from build123d import *

# Parameters (mm, degrees)
SALIENTE_EXTRUIR1_DEPTH = 2.5
CROQUIS2_W              = 5
CROQUIS2_H              = 12.7
SALIENTE_EXTRUIR2_DEPTH = 6.350000000000001
CORTAR_EXTRUIR1_REACH   = 52.655
CORTAR_EXTRUIR2_REACH   = 52.655
MATRIZC7_COUNT          = 3
REDONDEO3_R             = 3
REDONDEO4_R             = 3
REDONDEO5_R             = 3
REDONDEO6_R             = 3
REDONDEO7_R             = 3
REDONDEO8_R             = 3


with BuildPart() as part:
    # Croquis1 → Saliente-Extruir1 (new, symmetric)
    with BuildSketch(Plane(origin=(0, 0, 0), x_dir=(1, 0, 0), z_dir=(0, 1, 0))):
        with BuildLine():
            Line((-2.5, 28.650000000000002), (2.5, 28.650000000000002))
            Line((2.5, 28.650000000000002), (2.5, 20.849364905389077))
            ThreePointArc((2.5, 20.849364905389077), (2.8407417371092976, 18.26117445436386), (3.8397459621556003, 15.84936490538906))
            Line((3.8397459621556003, 15.84936490538906), (15.64582562299427, -4.599364905389191))
            ThreePointArc((15.64582562299427, -4.599364905389191), (17.235011848973173, -6.670432717254639), (19.306079660838602, -8.259618943233573))
            Line((19.306079660838602, -8.259618943233573), (26.061627818424082, -12.159936490539094))
            Line((26.061627818424082, -12.159936490539094), (23.561627818424125, -16.490063509461137))
            Line((23.561627818424125, -16.490063509461137), (16.806079660838638, -12.589745962155668))
            ThreePointArc((16.806079660838638, -12.589745962155668), (14.394270111863824, -11.590741737109344), (11.80607966083859, -11.25000000000002))
            Line((11.80607966083859, -11.25000000000002), (-11.806079660838877, -11.250000000000021))
            ThreePointArc((-11.806079660838877, -11.250000000000021), (-14.394270111864046, -11.590741737109328), (-16.806079660838808, -12.589745962155595))
            Line((-16.806079660838808, -12.589745962155595), (-23.561627818424295, -16.490063509460935))
            Line((-23.561627818424295, -16.490063509460935), (-26.061627818424316, -12.15993649053858))
            Line((-26.061627818424316, -12.15993649053858), (-19.30607966083857, -8.259618943233107))
            ThreePointArc((-19.30607966083857, -8.259618943233107), (-17.235011848973045, -6.670432717254254), (-15.645825622994131, -4.5993649053887635))
            Line((-15.645825622994131, -4.5993649053887635), (-3.8397459621555967, 15.849364905389269))
            ThreePointArc((-3.8397459621555967, 15.849364905389269), (-2.8407417371093064, 18.26117445436405), (-2.5000000000000004, 20.84936490538924))
            Line((-2.5000000000000004, 20.84936490538924), (-2.5, 28.650000000000002))
        make_face()
        with BuildLine():
            Line((4.999999999999967, -1.648e-14), (8.325317547305488, -1.919872981077918))
            Line((8.325317547305488, -1.919872981077918), (2.5, 8.169872981077836))
            Line((2.5, 8.169872981077836), (2.5000000000000004, 4.330127018922162))
            ThreePointArc((2.5000000000000004, 4.330127018922162), (3.16987298107781, 1.8301270189221883), (4.999999999999967, -1.648e-14))
        make_face(mode=Mode.SUBTRACT)
        with BuildLine():
            Line((-2.499999999999762, -4.330127018922147), (-5.825317547305628, -6.250000000000082))
            Line((-5.825317547305628, -6.250000000000082), (5.825317547305489, -6.249999999999961))
            Line((5.825317547305489, -6.249999999999961), (2.5000000000002185, -4.3301270189221945))
            ThreePointArc((2.5000000000002185, -4.3301270189221945), (1.9836e-13, -3.660254037844239), (-2.499999999999762, -4.330127018922147))
        make_face(mode=Mode.SUBTRACT)
        with BuildLine():
            Line((-2.5000000000000004, 4.330127018922227), (-2.5, 8.169872981077782))
            Line((-2.5, 8.169872981077782), (-8.325317547305644, -1.9198729810777775))
            Line((-8.325317547305644, -1.9198729810777775), (-5.000000000000053, 0))
            ThreePointArc((-5.000000000000053, 0), (-3.1698729810778152, 1.8301270189221972), (-2.5000000000000004, 4.330127018922227))
        make_face(mode=Mode.SUBTRACT)
    extrude(amount=SALIENTE_EXTRUIR1_DEPTH, both=True)

    # Croquis2 → Saliente-Extruir2 (add, symmetric)
    with BuildSketch(Plane(origin=(0, 0, 0), x_dir=(1, 0, 0), z_dir=(0, 1, 0))):
        with Locations((0, 35)):
            Rectangle(CROQUIS2_W, CROQUIS2_H)
    saliente_extruir2 = extrude(amount=SALIENTE_EXTRUIR2_DEPTH, both=True)

    # Croquis3 → Cortar-Extruir1 (cut, up to next)
    with BuildSketch(Plane(origin=(2.5, 0, 0), x_dir=(0, 0, -1), z_dir=(1, 0, 0)), mode=Mode.PRIVATE) as cortar_extruir1_sk1:
        with BuildLine():
            Line((32.754935969732706, 2.2450640302672804), (35, 4.490128060534589))
            Line((35, 4.490128060534589), (37.245064030267294, 2.245064030267292))
            ThreePointArc((37.245064030267294, 2.245064030267292), (35.00000000000001, -3.174999999999998), (32.754935969732706, 2.2450640302672804))
        make_face()
    cortar_extruir1_tool1 = extrude(cortar_extruir1_sk1.sketch, amount=-CORTAR_EXTRUIR1_REACH, mode=Mode.PRIVATE) & part.part
    cortar_extruir1 = cortar_extruir1_tool1.solids().sort_by_distance((2.5, 0.222977, -35))[0]
    add(cortar_extruir1, mode=Mode.SUBTRACT)

    # Croquis4 → Cortar-Extruir2 (cut, up to next)
    with BuildSketch(Plane.ZY.offset(2.5000000000000018), mode=Mode.PRIVATE) as cortar_extruir2_sk1:
        with BuildLine():
            Line((-41.35, 6.350000000000001), (-37.50000000000001, 6.350000000000001))
            ThreePointArc((-37.50000000000001, 6.350000000000001), (-40.22236110756822, 5.222361107568213), (-41.35, 2.500000000000002))
            Line((-41.35, 2.500000000000002), (-41.35, 6.350000000000001))
        make_face()
    cortar_extruir2_tool1 = extrude(cortar_extruir2_sk1.sketch, amount=-CORTAR_EXTRUIR2_REACH, mode=Mode.PRIVATE) & part.part
    # Croquis4 → Cortar-Extruir2 (cut, up to next)
    with BuildSketch(Plane.ZY.offset(2.5000000000000018), mode=Mode.PRIVATE) as cortar_extruir2_sk2:
        with BuildLine():
            Line((-32.5, 6.350000000000001), (-28.650000000000002, 6.350000000000001))
            Line((-28.650000000000002, 6.350000000000001), (-28.650000000000002, 2.5))
            ThreePointArc((-28.650000000000002, 2.5), (-29.777638892431792, 5.222361107568209), (-32.5, 6.350000000000001))
        make_face()
    cortar_extruir2_tool2 = extrude(cortar_extruir2_sk2.sketch, amount=-CORTAR_EXTRUIR2_REACH, mode=Mode.PRIVATE) & part.part
    # Croquis4 → Cortar-Extruir2 (cut, up to next)
    with BuildSketch(Plane.ZY.offset(2.5000000000000018), mode=Mode.PRIVATE) as cortar_extruir2_sk3:
        with BuildLine():
            Line((-41.35, -2.500000000000002), (-41.35, -6.350000000000001))
            Line((-41.35, -6.350000000000001), (-37.50000000000001, -6.350000000000001))
            ThreePointArc((-37.50000000000001, -6.350000000000001), (-40.22236110756821, -5.222361107568203), (-41.35, -2.500000000000002))
        make_face()
    cortar_extruir2_tool3 = extrude(cortar_extruir2_sk3.sketch, amount=-CORTAR_EXTRUIR2_REACH, mode=Mode.PRIVATE) & part.part
    # Croquis4 → Cortar-Extruir2 (cut, up to next)
    with BuildSketch(Plane.ZY.offset(2.5000000000000018), mode=Mode.PRIVATE) as cortar_extruir2_sk4:
        with BuildLine():
            Line((-28.650000000000002, -2.5000000000000004), (-28.650000000000002, -6.350000000000001))
            Line((-28.650000000000002, -6.350000000000001), (-32.5, -6.350000000000001))
            ThreePointArc((-32.5, -6.350000000000001), (-29.777638892431792, -5.222361107568209), (-28.650000000000002, -2.5000000000000004))
        make_face()
    cortar_extruir2_tool4 = extrude(cortar_extruir2_sk4.sketch, amount=-CORTAR_EXTRUIR2_REACH, mode=Mode.PRIVATE) & part.part
    cortar_extruir2_1 = cortar_extruir2_tool1.solids().sort_by_distance((-2.5, 5.490033, -40.490033))[0]
    add(cortar_extruir2_1, mode=Mode.SUBTRACT)
    cortar_extruir2_2 = cortar_extruir2_tool2.solids().sort_by_distance((-2.5, 5.490033, -29.509967))[0]
    add(cortar_extruir2_2, mode=Mode.SUBTRACT)
    cortar_extruir2_3 = cortar_extruir2_tool3.solids().sort_by_distance((-2.5, -5.490033, -40.490033))[0]
    add(cortar_extruir2_3, mode=Mode.SUBTRACT)
    cortar_extruir2_4 = cortar_extruir2_tool4.solids().sort_by_distance((-2.5, -5.490033, -29.509967))[0]
    add(cortar_extruir2_4, mode=Mode.SUBTRACT)
    cortar_extruir2 = cortar_extruir2_1 + cortar_extruir2_2 + cortar_extruir2_3 + cortar_extruir2_4  # Cortar-Extruir2 as one shape, for the pattern or mirror that repeats it

    # MatrizC7: Saliente-Extruir2, Cortar-Extruir1, Cortar-Extruir2 ×3 about axis
    matrizc7_axis = Axis((-4.13e-15, 0, 3.06e-15), (0, 1, 0))
    add([saliente_extruir2.rotate(matrizc7_axis, i * 360 / MATRIZC7_COUNT) for i in range(1, MATRIZC7_COUNT)])
    add([cortar_extruir1.rotate(matrizc7_axis, i * 360 / MATRIZC7_COUNT) for i in range(1, MATRIZC7_COUNT)], mode=Mode.SUBTRACT)
    add([cortar_extruir2.rotate(matrizc7_axis, i * 360 / MATRIZC7_COUNT) for i in range(1, MATRIZC7_COUNT)], mode=Mode.SUBTRACT)

    # Redondeo3
    redondeo3_edges = [part.edges().sort_by_distance(p)[0] for p in [
        (0, 2.5, -28.650000000000002),
    ]]
    fillet(redondeo3_edges, radius=REDONDEO3_R)

    # Redondeo4
    redondeo4_edges = [part.edges().sort_by_distance(p)[0] for p in [
        (-24.811627818424306, 2.5, 14.324999999999758),
    ]]
    fillet(redondeo4_edges, radius=REDONDEO4_R)

    # Redondeo5
    redondeo5_edges = [part.edges().sort_by_distance(p)[0] for p in [
        (24.811627818424103, 2.5, 14.325000000000117),
    ]]
    fillet(redondeo5_edges, radius=REDONDEO5_R)

    # Redondeo6
    redondeo6_edges = [part.edges().sort_by_distance(p)[0] for p in [
        (-24.811627818424306, -2.5, 14.324999999999758),
    ]]
    fillet(redondeo6_edges, radius=REDONDEO6_R)

    # Redondeo7
    redondeo7_edges = [part.edges().sort_by_distance(p)[0] for p in [
        (0, -2.5, -28.650000000000002),
    ]]
    fillet(redondeo7_edges, radius=REDONDEO7_R)

    # Redondeo8
    redondeo8_edges = [part.edges().sort_by_distance(p)[0] for p in [
        (24.811627818424103, -2.5, 14.325000000000117),
    ]]
    fillet(redondeo8_edges, radius=REDONDEO8_R)


solid = part.part
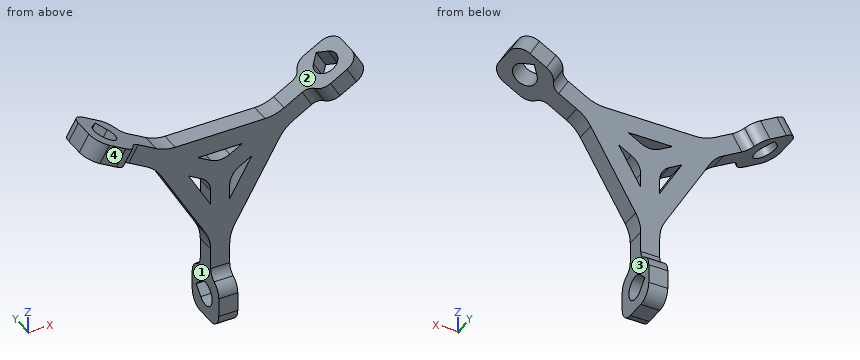
Geometry check sheet. Reference: the model listing, model coordinates, mm. Face numbers are marked on the shaded views. Round coordinates to 2 decimals unless told otherwise and drop trailing zeros. Write each loop counter-clockwise with the first axis right and the second up, starting at its lowest first coordinate (ties: lowest second). Pieces come first, ordered by that corner, then holes. Notation, with made-up numbers: (86.25, -39.5) -> (92.25, -39.5) arc R18 ccw to (92.25, -13.5) -> close; hole circle Ø5 at (-25.75, 52.25). An arc over 180 degrees is marked (long way). One line per item, written item: value. Start each with the question number.
(1) Draft check along X on the marked faces 1, 2, 3 and 4. Enter one of: +X half, -X half, draft (parallel to the pull), parting line (faces both ways), or undercut.
(2) Scan lines: line 1 (Z direction, x = -1.4, y = 0) (3 decimals); line 2 (Z direction, x = -0.4, y = 0) (3 decimals); line 3 (X direction, y = -2.5, z = 17). Record each from-to range of solid material in increasing order. Write a range as [from, to].
(3) Cross-section at A-A, the plane y = 0. Give the number of separate pieces and of enclosed holes in the cut face, and give its area (3 significant figures).
(4) Cross-section at B-B, the plane z = -18.5. Record the cut outline in (x, y).
(5) Go/stop test with flat-tipped pins: pin 1 Ø21 at (x, z) = (11.5, -15) entering from +Y; pin 2 Ø1.5 at (y, z) = (-1.5, -15.5) entering from -X; pin 3 Ø12.5 at (x, z) = (2, -6) entering from -Y; pin 4 Ø4 at (x, y) = (3, -1) entering from -Z. Record where each tip stops, or that it passes through.
Answer:
1. face 1: -X half
1. face 2: undercut
1. face 3: +X half
1. face 4: draft
2. line 1: [-41.35, -38.175], [-31.825, 3.86], [6.25, 11.25]
2. line 2: [-41.35, -38.175], [-31.825, 3.676], [6.25, 11.25]
2. line 3: [-34.44, -32.86], [-28.34, -24.44], [24.44, 28.34], [32.86, 34.44]
3. separate pieces: 4
3. enclosed holes: 3
3. area: 827 mm²
4. outline: (-2.78, -2.5) -> (2.78, -2.5) -> (2.78, 2.5) -> (-2.78, 2.5) -> close
5. pin 1: y = 2.5
5. pin 2: x = -4.47
5. pin 3: y = -2.5
5. pin 4: z = -41.35
